The model under review builds one solid part; all positions refer to its coordinate system, in mm. A direction names the side the tool comes from. Round coordinates to 2 decimals unless told otherwise and drop trailing zeros. Loops run counter-clockwise (first coordinate to the right, second up) from the corner with the lowest first, then second, coordinate; pieces in that order, holes last. Notation, with made-up numbers: M -19.5,-3.75 L -14.5,-3.75 A31 ccw -14.5,25.25 Z; hole C 70.5,79 d6. An arc over 180 degrees is marked long. Answer as a JSON object with one key per item and string values. Group by question number.
Item 1: Consider section A-A (y = 75.5). State how many separate pieces and enclosed holes the cut face has, and give its area (3 significant figures).
Item 2: The part is to be moulded in two halves that separate along Y. For faces 3 (the face through (136.56, 107.81, 1.57)), 4 (the face through (151.45, 7.26, 1.61)), 5 (the face through (127.478, 117.958, 1.61)), say which applies: +Y half, -Y half, draft (parallel to the pull), parting line (faces both ways), or undercut.
Item 3: Insertion check: P1, Ø3, axis at x = 107.95, y = 139.7, coming from the -Z side. The pin has a flat end and moves straight along its axis. Give the tip position at first contact, or say it passes through.
Item 4: Consider section B-B (x = 57.15). Give the boundary of the cut face in (y, z) (3 decimals), and give its area (3 significant figures).
Item 5: Tool access review of faces 1 (the face through (133.218, 84.845, 1.565)), 2 (the face through (95, 171.45, 2)): name each direction out of +Z, -Z, +X, -X, +Y, -Y from which nothing blocks a thin tool from reaching the whole face with its end or side.
Item 6: To check wall thickness, follow line 1 (X direction, y = 165.1, z = 2); line 2 (X direction, y = 152.5, z = 1.2); line 3 (X direction, y = 61.5, z = 0.5). State the ranges of each line that lie inside material, in increasing order.
```python
from build123d import *

# Parameters (mm, degrees)
SKETCH1_R           = 2.4892
BOSS_EXTRUDE1_DEPTH = 3.175
CUT_EXTRUDE1_DEPTH  = 4.175
FILLET1_R           = 3.175
FILLET1_2_R         = 1.5875
FILLET2_R           = 3.175


with BuildPart() as part:
    # Sketch1 → Boss-Extrude1 (new body)
    with BuildSketch(Plane.XY):
        Polygon((38.1, 44.45), (69.85, 171.45), (120.65, 171.45), (152.4, 44.45), (152.4, 6.35), (38.1, 6.35), align=None)
        with Locations((44.45, 38.1)):
            Circle(SKETCH1_R, mode=Mode.SUBTRACT)
        with Locations((57.15, 38.1)):
            Circle(SKETCH1_R, mode=Mode.SUBTRACT)
        with Locations((69.85, 38.1)):
            Circle(SKETCH1_R, mode=Mode.SUBTRACT)
        with Locations((82.55, 38.1)):
            Circle(SKETCH1_R, mode=Mode.SUBTRACT)
        with Locations((95.25, 38.1)):
            Circle(SKETCH1_R, mode=Mode.SUBTRACT)
        with Locations((107.95, 38.1)):
            Circle(SKETCH1_R, mode=Mode.SUBTRACT)
        with Locations((120.65, 38.1)):
            Circle(SKETCH1_R, mode=Mode.SUBTRACT)
        with Locations((133.35, 38.1)):
            Circle(SKETCH1_R, mode=Mode.SUBTRACT)
        with Locations((146.05, 38.1)):
            Circle(SKETCH1_R, mode=Mode.SUBTRACT)
        with Locations((44.45, 25.4)):
            Circle(SKETCH1_R, mode=Mode.SUBTRACT)
        with Locations((57.15, 25.4)):
            Circle(SKETCH1_R, mode=Mode.SUBTRACT)
        with Locations((69.85, 25.4)):
            Circle(SKETCH1_R, mode=Mode.SUBTRACT)
        with Locations((82.55, 25.4)):
            Circle(SKETCH1_R, mode=Mode.SUBTRACT)
        with Locations((95.25, 25.4)):
            Circle(SKETCH1_R, mode=Mode.SUBTRACT)
        with Locations((107.95, 25.4)):
            Circle(SKETCH1_R, mode=Mode.SUBTRACT)
        with Locations((120.65, 25.4)):
            Circle(SKETCH1_R, mode=Mode.SUBTRACT)
        with Locations((133.35, 25.4)):
            Circle(SKETCH1_R, mode=Mode.SUBTRACT)
        with Locations((146.05, 25.4)):
            Circle(SKETCH1_R, mode=Mode.SUBTRACT)
        with Locations((44.45, 12.7)):
            Circle(SKETCH1_R, mode=Mode.SUBTRACT)
        with Locations((57.15, 12.7)):
            Circle(SKETCH1_R, mode=Mode.SUBTRACT)
        with Locations((69.85, 12.7)):
            Circle(SKETCH1_R, mode=Mode.SUBTRACT)
        with Locations((82.55, 12.7)):
            Circle(SKETCH1_R, mode=Mode.SUBTRACT)
        with Locations((95.25, 12.7)):
            Circle(SKETCH1_R, mode=Mode.SUBTRACT)
        with Locations((107.95, 12.7)):
            Circle(SKETCH1_R, mode=Mode.SUBTRACT)
        with Locations((120.65, 12.7)):
            Circle(SKETCH1_R, mode=Mode.SUBTRACT)
        with Locations((133.35, 12.7)):
            Circle(SKETCH1_R, mode=Mode.SUBTRACT)
        with Locations((146.05, 12.7)):
            Circle(SKETCH1_R, mode=Mode.SUBTRACT)
        with Locations((82.55, 88.9)):
            Circle(SKETCH1_R, mode=Mode.SUBTRACT)
        with Locations((95.25, 88.9)):
            Circle(SKETCH1_R, mode=Mode.SUBTRACT)
        with Locations((107.95, 88.9)):
            Circle(SKETCH1_R, mode=Mode.SUBTRACT)
        with Locations((95.25, 101.6)):
            Circle(SKETCH1_R, mode=Mode.SUBTRACT)
        with Locations((107.95, 101.6)):
            Circle(SKETCH1_R, mode=Mode.SUBTRACT)
        with Locations((95.25, 114.3)):
            Circle(SKETCH1_R, mode=Mode.SUBTRACT)
        with Locations((107.95, 114.3)):
            Circle(SKETCH1_R, mode=Mode.SUBTRACT)
        with Locations((95.25, 127)):
            Circle(SKETCH1_R, mode=Mode.SUBTRACT)
        with Locations((107.95, 127)):
            Circle(SKETCH1_R, mode=Mode.SUBTRACT)
        with Locations((95.25, 139.7)):
            Circle(SKETCH1_R, mode=Mode.SUBTRACT)
        with Locations((107.95, 139.7)):
            Circle(SKETCH1_R, mode=Mode.SUBTRACT)
        with Locations((95.25, 152.4)):
            Circle(SKETCH1_R, mode=Mode.SUBTRACT)
        with Locations((107.95, 152.4)):
            Circle(SKETCH1_R, mode=Mode.SUBTRACT)
        with Locations((95.25, 165.1)):
            Circle(SKETCH1_R, mode=Mode.SUBTRACT)
        with Locations((107.95, 165.1)):
            Circle(SKETCH1_R, mode=Mode.SUBTRACT)
        with Locations((82.55, 101.6)):
            Circle(SKETCH1_R, mode=Mode.SUBTRACT)
        with Locations((82.55, 114.3)):
            Circle(SKETCH1_R, mode=Mode.SUBTRACT)
        with Locations((82.55, 127)):
            Circle(SKETCH1_R, mode=Mode.SUBTRACT)
        with Locations((82.55, 139.7)):
            Circle(SKETCH1_R, mode=Mode.SUBTRACT)
        with Locations((82.55, 152.4)):
            Circle(SKETCH1_R, mode=Mode.SUBTRACT)
        with Locations((82.55, 165.1)):
            Circle(SKETCH1_R, mode=Mode.SUBTRACT)
    extrude(amount=BOSS_EXTRUDE1_DEPTH)

    # Sketch2 → Cut-Extrude1 (cut, through all)
    with BuildSketch(Plane.XY.offset(3.175)):
        Polygon((46.232930181, 50.8), (68.213642455, 50.8), (57.223286318, 94.761424548), align=None)
        Polygon((69.85, 96.446639639), (60.074697636, 96.446639639), (69.85, 57.345430181), align=None)
        Polygon((58.43834009, 99.621639639), (69.85, 99.621639639), (69.85, 145.268279277), align=None)
        Polygon((120.65, 99.621639639), (132.06165991, 99.621639639), (120.65, 145.268279277), align=None)
        Polygon((120.65, 96.446639639), (120.65, 57.345430181), (130.425302364, 96.446639639), align=None)
        Polygon((122.286357545, 50.8), (144.267069819, 50.8), (133.276713682, 94.761424548), align=None)
    extrude(amount=-CUT_EXTRUDE1_DEPTH, mode=Mode.SUBTRACT)

    # Fillet1
    fillet1_edges = [part.edges().sort_by_distance(p)[0] for p in [
        (46.232930181, 50.8, 1.5875),
        (57.223286318, 94.761424548, 1.5875),
        (68.213642455, 50.8, 1.5875),
        (60.074697636, 96.446639639, 1.5875),
        (69.85, 96.446639639, 1.5875),
        (69.85, 99.621639639, 1.5875),
        (58.43834009, 99.621639639, 1.5875),
        (120.65, 57.345430181, 1.5875),
        (132.06165991, 99.621639639, 1.5875),
        (120.65, 99.621639639, 1.5875),
        (120.65, 96.446639639, 1.5875),
        (130.425302364, 96.446639639, 1.5875),
        (133.276713682, 94.761424548, 1.5875),
        (122.286357545, 50.8, 1.5875),
        (144.267069819, 50.8, 1.5875),
    ]]
    fillet(fillet1_edges, radius=FILLET1_R)

    # Fillet1 2
    fillet1_2_edges = [part.edges().sort_by_distance(p)[0] for p in [
        (69.85, 145.268279277, 1.5875),
        (69.85, 57.345430181, 1.5875),
        (120.65, 145.268279277, 1.5875),
    ]]
    fillet(fillet1_2_edges, radius=FILLET1_2_R)

    # Fillet2
    fillet2_edges = [part.edges().sort_by_distance(p)[0] for p in [
        (152.4, 44.45, 1.5875),
        (152.4, 6.35, 1.5875),
        (38.1, 6.35, 1.5875),
        (38.1, 44.45, 1.5875),
        (69.85, 171.45, 1.5875),
        (120.65, 171.45, 1.5875),
    ]]
    fillet(fillet2_edges, radius=FILLET2_R)


solid = part.part
```
Geometry results:
{
 "1": {"separate pieces": "4", "enclosed holes": "0", "area": "238 mm^2"},
 "2": {"face 3": "+Y half", "face 4": "-Y half", "face 5": "undercut"},
 "3": {"P1": "passes through"},
 "4": {"outline": "M 6.35,0 L 10.211,0 L 10.211,3.175 L 6.35,3.175 Z; M 15.189,0 L 22.911,0 L 22.911,3.175 L 15.189,3.175 Z; M 27.889,0 L 35.611,0 L 35.611,3.175 L 27.889,3.175 Z; M 40.589,0 L 50.8,0 L 50.8,3.175 L 40.589,3.175 Z; M 84.845,0 L 120.65,0 L 120.65,3.175 L 84.845,3.175 Z", "area": "207 mm^2"},
 "5": {"face 1": "+Z, -Z", "face 2": "+Z, -Z, +X, -X, +Y"},
 "6": {"line 1": "x = 68.26 to 80.06, 85.04 to 92.76, 97.74 to 105.46, 110.44 to 122.24", "line 2": "x = 65.11 to 80.06, 85.04 to 92.76, 97.74 to 105.46, 110.44 to 125.39", "line 3": "x = 42.36 to 48.91, 65.54 to 124.96, 141.59 to 148.14"}
}
